```python
from build123d import *

# Parameters (mm, degrees)
SKETCH1_W               = 20
SKETCH1_H               = 20
BOSS_EXTRUDE1_DEPTH     = 7.5
SKETCH1_3_W             = 20
SKETCH1_3_H             = 20
CUT_EXTRUDE2_DEPTH      = 1.5
SKETCH3_W               = 10
SKETCH3_H               = 20
BOSS_EXTRUDE2_DEPTH     = 1.5
SKETCH4_R               = 1.5
CUT_EXTRUDE3_DEPTH      = 7.5
CUT_EXTRUDE4_DEPTH      = 17.007810594
CUT_EXTRUDE4_DEPTH_BACK = 17.007810594
SKETCH5_R               = 1.5


with BuildPart() as part:
    # Sketch1 → Boss-Extrude1 (new, symmetric)
    with BuildSketch(Plane(origin=(0, 0, 0), x_dir=(1, 0, 0), z_dir=(0, 1, 0))):
        Rectangle(SKETCH1_W, SKETCH1_H)
    extrude(amount=BOSS_EXTRUDE1_DEPTH, both=True)

    # Sketch1_3 → Cut-Extrude2 (cut, symmetric)
    with BuildSketch(Plane(origin=(0, 0, 0), x_dir=(1, 0, 0), z_dir=(0, 1, 0))):
        Rectangle(SKETCH1_3_W, SKETCH1_3_H)
    extrude(amount=CUT_EXTRUDE2_DEPTH, both=True, mode=Mode.SUBTRACT)


with BuildPart() as cut_extrude2_piece_1:
    # of the separate pieces the step leaves, piece 1, a body of its own (cut_extrude2_pieces)
    add(part.part.solids().sort_by_distance((-10, -7.5, -10))[0])



with BuildPart() as cut_extrude2_piece_2:
    # of the separate pieces the step leaves, piece 2, a body of its own (cut_extrude2_pieces)
    add(part.part.solids().sort_by_distance((-10, 1.5, -10))[0])


with BuildPart() as cut_extrude2_piece_1_1:
    add(cut_extrude2_piece_1.part)

    add(cut_extrude2_piece_2.part)  # Boss-Extrude2 merges Cut-Extrude2 piece 2
    # Sketch3 → Boss-Extrude2 (add, symmetric)
    with BuildSketch(Plane(origin=(0, 0, 0), x_dir=(1, 0, 0), z_dir=(0, 1, 0))):
        with Locations((5, 0)):
            Rectangle(SKETCH3_W, SKETCH3_H)
    extrude(amount=BOSS_EXTRUDE2_DEPTH, both=True)

    # Sketch4 → Cut-Extrude3 (cut)
    with BuildSketch(Plane(origin=(10, 0, 0), x_dir=(0, 0, -1), z_dir=(1, 0, 0))):
        Circle(SKETCH4_R)
    extrude(amount=-CUT_EXTRUDE3_DEPTH, mode=Mode.SUBTRACT)

    # Sketch5 → Cut-Extrude4 (cut, two sides: drawn at the far end of the back side and taken through both)
    with BuildSketch(Plane(origin=(0, 0, 0), x_dir=(1, 0, 0), z_dir=(0, 1, 0)).offset(-CUT_EXTRUDE4_DEPTH_BACK)):
        with Locations(Location((-6, 6, 0), (0, 0, 270))):
            Circle(SKETCH5_R)
        with Locations(Location((6, 6, 0), (0, 0, 270))):
            Circle(SKETCH5_R)
        with Locations(Location((6, -6, 0), (0, 0, 270))):
            Circle(SKETCH5_R)
        with Locations(Location((-6, -6, 0), (0, 0, 270))):
            Circle(SKETCH5_R)
    extrude(amount=CUT_EXTRUDE4_DEPTH + CUT_EXTRUDE4_DEPTH_BACK, mode=Mode.SUBTRACT)


solid = cut_extrude2_piece_1_1.part
```
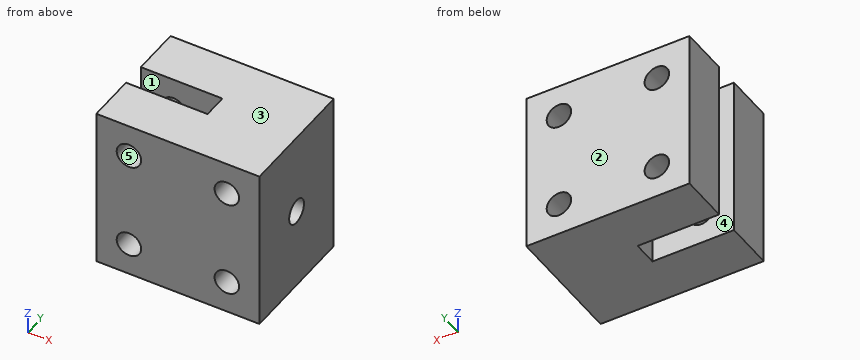
Source: CAD feature listing. Evaluate the final solid. Frame: model axes, mm. Face numbers are marked on the shaded views. A direction names the side the tool comes from. Give positions to 0.01 mm unless a question says otherwise; leave off trailing zeros. Order: outer loops, then holes, each group sorted by start corner. A loop starts at its lowest first (then second) coordinate and runs counter-clockwise, first axis right, second up.
(1) Material intervals for line 1 along X through (y, z) = (6.15, 6); line 2 along Y through (x, z) = (-8.75, 5.25), sorted ascending.
(2) Access query for the marked faces 4 and 5. Directions: +Z, -Z, +X, -X, +Y, -Y. A direction counts if a zero-diameter tool reaches every point of the face in a straight line with its end or side. Return the directions, or none.
(3) Section query A-A (z = 6). Return the cut outline in (x, y), plus the area to 3 significant figures.
(4) Section query D-D (z = 8.75). Return the cut outline in (x, y).
(5) Section query B-B (y = 5). Return the cut outline in (x, z).
(6) Pull-direction query (Y, two-part tool) for the marked faces 1, 2 and 3; classes: +Y half, -Y half, draft (parallel to the pull), parting line (faces both ways), or undercut.
(7) Section query C-C (x = -3.75). Return the cut outline in (y, z).
(8) Contact query for a flat-ended pin moving along its axis: P1, Ø2.5, axis at y = 0, z = 0, coming from the -X side. Output: stop coordinate, or through.
Outcome:
1. line 1: x = -10 to -7.5, -4.5 to 4.5, 7.5 to 10
1. line 2: y = -7.5 to -1.5, 1.5 to 7.5
2. face 4: +Z, -Z, -X
2. face 5: +Y, -Y
3. outline: (-10, -7.5) - (-7.5, -7.5) - (-7.5, -1.5) - (-10, -1.5) - close; (-10, 1.5) - (-7.5, 1.5) - (-7.5, 7.5) - (-10, 7.5) - close; (-4.5, -7.5) - (4.5, -7.5) - (4.5, 7.5) - (-4.5, 7.5) - (-4.5, 1.5) - (0, 1.5) - (0, -1.5) - (-4.5, -1.5) - close; (7.5, -7.5) - (10, -7.5) - (10, 7.5) - (7.5, 7.5) - close
3. area: 189 mm2
4. outline: (-10, -7.5) - (10, -7.5) - (10, 7.5) - (-10, 7.5) - (-10, 1.5) - (0, 1.5) - (0, -1.5) - (-10, -1.5) - close
5. outline: (-10, -10) - (10, -10) - (10, 10) - (-10, 10) - close; hole circle Ø3 at (-6, -6); hole circle Ø3 at (-6, 6); hole circle Ø3 at (6, -6); hole circle Ø3 at (6, 6)
6. face 1: undercut
6. face 2: +Y half
6. face 3: draft
7. outline: (-7.5, -10) - (-1.5, -10) - (-1.5, 10) - (-7.5, 10) - close; (1.5, -10) - (7.5, -10) - (7.5, 10) - (1.5, 10) - close
8. P1: stops at x = 0
